```python
from build123d import *

# Parameters (mm, degrees)
F1_DEPTH = 50
F2_T     = -2.54


with BuildPart() as f1:
    # F0 (on Top) → F1 (new body)
    with BuildSketch(Plane.XY):
        Polygon((14.849242, -14.849242), (0, 0), (-14.849242, -14.849242), align=None)
    extrude(amount=F1_DEPTH)

    # F2
    f2_openings = [f1.faces().sort_by_distance(p)[0] for p in [
        (-7.424621, -7.424621, 25),
        (7.424621, -7.424621, 25),
    ]]
    offset(amount=F2_T, openings=f2_openings)


solid = f1.part
```
Work out the finished part from the listing and answer in its coordinate system (mm). A direction names the side the tool comes from. Give positions to 0.01 mm unless a question says otherwise; leave off trailing zeros. Loops run counter-clockwise (first coordinate to the right, second up) from the corner with the lowest first, then second, coordinate; pieces in that order, holes last. Notation, with made-up numbers: (-11, 58) -> (41, 58) arc R18 cw to (41, 75) -> close; hole circle Ø11 at (-26.5, 14). An arc over 180 degrees is marked (long way). Use CSV: the item, a comma, the result in double quotes.
1. The part is cut by section C-C (z = 8). Write down the section's boundary in (x, y).
Found:
outline,"(-14.85, -14.85) -> (14.85, -14.85) -> (12.31, -12.31) -> (-12.31, -12.31) -> close"
2. Flat-ended cylindrical pins translate along their axes: pin 1 Ø4 at (y, z) = (-11.5, 13.5) entering from +X; pin 2 Ø1.5 at (x, z) = (-0.5, 27) entering from +Y; pin 3 Ø5 at (y, z) = (-10, 41) entering from -X. Find the tip coordinate at first contact, or state that the pin passes through.
Found:
pin 1,"x = 13.5"
pin 2,"y = -12.31"
pin 3,"x = -12.5"
3. The part is cut by section D-D (x = 9.75). Write down the section's boundary in (y, z), then the cut area to 3 significant figures.
Found:
outline,"(-14.85, 0) -> (-9.75, 0) -> (-9.75, 2.54) -> (-12.31, 2.54) -> (-12.31, 47.46) -> (-9.75, 47.46) -> (-9.75, 50) -> (-14.85, 50) -> close"
area,"140 mm^2"
4. A tool of negligible diameter and unlimited length cuts with its end or side. For faces 4 (the flat face through (0, -12.309, 25)), 5 (the flat face through (13, -13, 17)), from which of +Z, -Z, +X, -X, +Y, -Y can it reach the whole face along a straight path? Write none if from no direction.
Found:
face 4,"+X, -X, +Y"
face 5,"+Z, -Z, +X, +Y"
5. The part is cut by section A-A (y = -2). Write down the section's boundary in (x, z), then the cut area to 3 significant figures.
Found:
outline,"(-2, 0) -> (2, 0) -> (2, 2.54) -> (-2, 2.54) -> close; (-2, 47.46) -> (2, 47.46) -> (2, 50) -> (-2, 50) -> close"
area,"20.3 mm^2"
6. The mould has two halves that part along Z. Classify faces 1 (the flat face through (0, -14.849, 25)), 2 (the flat face through (0, -9, 0)), 3 (the flat face through (0, -7, 47.46)): +Z half, -Z half, draft (parallel to the pull), parting line (faces both ways), or undercut.
Found:
face 1,"draft"
face 2,"-Z half"
face 3,"undercut"
7. The part is cut by section B-B (x = 6.5). Write down the section's boundary in (y, z).
Found:
outline,"(-14.85, 0) -> (-6.5, 0) -> (-6.5, 2.54) -> (-12.31, 2.54) -> (-12.31, 47.46) -> (-6.5, 47.46) -> (-6.5, 50) -> (-14.85, 50) -> close"
8. Straight lines are drawn through the part: line 1 (Z direction, x = 5.25, y = -8.25); line 2 (Y direction, x = -1.75, z = 42); line 3 (X direction, y = -12.75, z = 47). For each, find the intervals that lie inside material, in ascending order.
Found:
line 1,"0 to 2.54, 47.46 to 50"
line 2,"-14.85 to -12.31"
line 3,"-12.75 to 12.75"
